Part model, mm, in its own coordinate system. A direction names the side the tool comes from. Coordinates: 2 decimals unless noted, no trailing zeros. Write each loop counter-clockwise with the first axis right and the second up, starting at its lowest first coordinate (ties: lowest second). Pieces come first, ordered by that corner, then holes. Notation, with made-up numbers: (-3, 83) -> (15, 83) arc R11 cw to (15, 96) -> close; hole circle Ø9 at (68, -2). An arc over 180 degrees is marked (long way). Write item = value, one per line. Start each with the question number.
Q1. Pull direction X, two halves, no side cores. Call faces 3 (the flat face through (3.014, -1.839, 1.479)), 4 (the flat face through (-7.4, 4.5, 1.5)), 5 (the flat face through (7.605, 4.148, 1.479)): released by +X, released by -X, zero draft, split by the parting line, or undercut.
Q2. Band-saw the part on B-B, the plane z = 1.75. List the corners of the cut face in (x, y), plus the area to 3 significant figures.
Q3. Tool access for faces 1 (the flat face through (0, -8.66, 1)), 2 (the flat face through (-3.1, -1.69, 1.48)): list every direction of +Z, -Z, +X, -X, +Y, -Y with a clear straight run to the whole face (end or side of a thin tool).
Q4. Probe line 1 (Y direction, x = 5, z = 2.5); line 2 (X direction, y = 3, z = 0.75); line 3 (Y direction, x = -0.5, z = 1.85). List the from-to ranges inside material, lowest first.
Q5. Band-saw the part on A-A, the plane y = -5.5. List the corners of the cut face in (x, z), plus the area to 3 significant figures.
Q6. Pin check, flat tips, straight feed: P1, Ø1.5, axis at y = -5.5, z = 2, coming from the -X side; P2, Ø1, axis at x = -1.5, z = 2.5, coming from the +Y side. Stop position of each tip, or through.
Q7. Band-saw the part on D-D, the plane y = 8.75. List the corners of the cut face in (x, z), plus the area to 3 significant figures.
Q8. Band-saw the part on C-C, the plane x = -3. List the corners of the cut face in (y, z), plus the area to 3 significant figures.
from build123d import *

# Parameters (mm, degrees)
F1_DEPTH = 1.5
F4_DEPTH = 1.5
F5_DEPTH = 1.5


with BuildPart() as f1:
    # F0 (on Top) → F1 (new body)
    with BuildSketch(Plane.XY):
        Polygon((-15, -8.6602540378), (15, -8.6602540378), (0, 17.3205080757), align=None)
    extrude(amount=F1_DEPTH)

    # F3 (on face) → F4 (cut)
    with BuildSketch(Plane.XY.offset(1.5)):
        Polygon((0, -7.0602540378), (6.1143593539, 3.5301270189), (-6.1143593539, 3.5301270189), align=None)
    extrude(amount=-F4_DEPTH, mode=Mode.SUBTRACT)

    # F5 (add): a face of the model
    f5_faces = [f1.faces().sort_by_distance(p)[0] for p in [
        (-7.1563068229, 4.1316956706, 1.5),
    ]]
    extrude(f5_faces, amount=F5_DEPTH)


solid = f1.part
Ans:
q1.face_3 = undercut
q1.face_4 = released by -X
q1.face_5 = released by +X
q2.outline = (-15, -8.66) -> (15, -8.66) -> (0, 17.32) -> close; hole (-6.11, 3.53) -> (0, -7.06) -> (6.11, 3.53) -> close
q2.area = 325 mm2
q3.face_1 = +Z, -Z, +X, -X, -Y
q3.face_2 = +Z, -Z
q4.line_1 = -8.66 to 1.6, 3.53 to 8.66
q4.line_2 = -8.27 to -5.81, 5.81 to 8.27
q4.line_3 = -8.66 to -6.19, 3.53 to 16.45
q5.outline = (-13.18, 0) -> (-0.9, 0) -> (-0.9, 3) -> (-13.18, 3) -> close; (0.9, 0) -> (13.18, 0) -> (13.18, 3) -> (0.9, 3) -> close
q5.area = 73.6 mm2
q6.P1 = -13.61
q6.P2 = 15.59
q7.outline = (-4.95, 0) -> (4.95, 0) -> (4.95, 3) -> (-4.95, 3) -> close
q7.area = 29.7 mm2
q8.outline = (-8.66, 0) -> (-1.86, 0) -> (-1.86, 3) -> (-8.66, 3) -> close; (3.53, 0) -> (12.12, 0) -> (12.12, 3) -> (3.53, 3) -> close
q8.area = 46.2 mm2
